```python
from build123d import *

# Parameters (mm, degrees)
F0_W     = 59.3015290797
F0_H     = 91.5408506989
F1_DEPTH = 47.752
F2_R     = 16.5566766108
F3_T     = -2.54


# Not quite as in the source:
# - a shell that OpenCascade refuses in one call is made with other operations: the cavity is built on its own and cut out


with BuildPart() as f1:
    # F0 (on Front) → F1 (new body)
    with BuildSketch(Plane.XZ):
        with Locations((-0.7059704512, -7.1773678064)):
            Rectangle(F0_W, F0_H)
    extrude(amount=F1_DEPTH)

    # F2
    f2_edges = [f1.edges().sort_by_distance(p)[0] for p in [
        (-30.356735, -23.876, 38.593058),
        (-30.356735, -23.876, -52.947793),
        (-30.356735, 0, -7.177368),
        (-30.356735, -47.752, -7.177368),
        (28.944794, -23.876, -52.947793),
        (-0.70597, 0, -52.947793),
        (-0.70597, -47.752, -52.947793),
        (28.944794, -23.876, 38.593058),
        (-0.70597, 0, 38.593058),
        (-0.70597, -47.752, 38.593058),
    ]]
    fillet(f2_edges, radius=F2_R)

    # F3: a shell. OpenCascade refuses it in one call, so the cavity is built on its own and cut out:
    # the body offset inwards by the wall thickness, plus a prism from it out through each open face.
    f3_core = offset(f1.part, amount=F3_T, mode=Mode.PRIVATE)
    f3_exits = [f3_core.faces().sort_by_distance(p)[0] for p in [
        (26.404794, -23.876, -7.177368),
    ]]
    add(f3_core, mode=Mode.SUBTRACT)
    extrude(f3_exits, amount=-F3_T, mode=Mode.SUBTRACT)


solid = f1.part
```
The model under review builds one solid part; all positions refer to its coordinate system, in mm. A direction names the side the tool comes from. Round coordinates to 2 decimals unless told otherwise and drop trailing zeros. Loops run counter-clockwise (first coordinate to the right, second up) from the corner with the lowest first, then second, coordinate; pieces in that order, holes last. Notation, with made-up numbers: M 57.5,-24 L 86.5,-24 A27 ccw 86.5,0 Z; hole C 32,-31 d3. An arc over 180 degrees is marked long. Put each result on its own line as item: value.
Q1. To check wall thickness, follow L1, parallel to Y at x = 12.5, z = 19; L2, parallel to Y at x = -4, z = -37; L3, parallel to Z at x = 17, y = -19. State the ranges of each line that lie inside material, in increasing order.
Result set:
L1: y = -47.75 to -45.21, -2.54 to 0
L2: y = -47.74 to -45.2, -2.55 to -0.01
L3: z = -52.29 to -49.63, 35.27 to 37.94
Q2. Machinability: for faces 4 (the flat face through (-30.357, -24, -8)), 5 (the flat face through (28, -24, -36.391)), 6 (the cylindrical face through (6.58, -41, -46.41)), which of the approach directions +Z, -Z, +X, -X, +Y, -Y give a long, thin tool a straight path to every point of the face, cutting with its end or side? Answer none if there is none.
Result set:
face 4: +Z, -Z, -X, +Y, -Y
face 5: +X
face 6: none
Q3. For pin 1 (21.5 mm diameter, centred on x = 12, z = -0.5, fed in from +Y); pin 2 (11.5 mm diameter, centred on y = -26.5, z = -4.5, fed in from +X); pin 3 (5 mm diameter, centred on x = -20.5, z = -15.5, fed in from +Y); pin 4 (1.5 mm diameter, centred on x = 9, y = -5.5, fed in from +Z), all flat-tipped, find the tip position at first contact; note any pin that passes through.
Result set:
pin 1: stops at y = 0
pin 2: stops at x = -27.78
pin 3: stops at y = -0.54
pin 4: stops at z = 34.99
Q4. Consider section B-B, the plane y = -29. Give the boundary of the cut face in (x, z).
Result set:
outline: M -30.36,-36.39 A16.56 ccw -13.8,-52.95 L 12.39,-52.95 A16.56 ccw 28.94,-36.39 L 26.4,-36.39 A14.02 cw 12.39,-50.41 L -13.8,-50.41 A14.02 cw -27.82,-36.39 L -27.82,22.04 A14.02 cw -13.8,36.05 L 12.39,36.05 A14.02 cw 26.4,22.04 L 28.94,22.04 A16.56 ccw 12.39,38.59 L -13.8,38.59 A16.56 ccw -30.36,22.04 Z
Q5. Consider section A-A, the plane z = 12. Give the boundary of the cut face in (x, y).
Result set:
outline: M -30.36,-31.2 A16.56 ccw -13.8,-47.75 L 28.94,-47.75 L 28.94,-45.21 L -13.8,-45.21 A14.02 cw -27.82,-31.2 L -27.82,-16.56 A14.02 cw -13.8,-2.54 L 28.94,-2.54 L 28.94,0 L -13.8,0 A16.56 ccw -30.36,-16.56 Z
Q6. Consider section D-D, the plane z = 32.5. Give the boundary of the cut face in (x, y).
Result set:
outline: M -26.63,-31.2 A12.83 ccw -13.8,-44.03 L 25.22,-44.03 L 25.22,-3.73 L -13.8,-3.73 A12.83 ccw -26.63,-16.56 Z; hole M -23.13,-31.2 A9.33 ccw -13.8,-40.52 L 21.71,-40.52 L 21.71,-7.23 L -13.8,-7.23 A9.33 ccw -23.13,-16.56 Z
Q7. Consider section C-C, the plane x = -8.5. Give the boundary of the cut face in (y, z).
Result set:
outline: M -47.75,-36.39 A16.56 ccw -31.2,-52.95 L -16.56,-52.95 A16.56 ccw 0,-36.39 L 0,22.04 A16.56 ccw -16.56,38.59 L -31.2,38.59 A16.56 ccw -47.75,22.04 Z; hole M -45.21,-36.39 A14.02 ccw -31.2,-50.41 L -16.56,-50.41 A14.02 ccw -2.54,-36.39 L -2.54,22.04 A14.02 ccw -16.56,36.05 L -31.2,36.05 A14.02 ccw -45.21,22.04 Z
Q8. Mouldability with a two-part tool opening along X and no side actions: class faces 1 (the cylindrical face through (6.6, -6.8, 32.1)), 2 (the flat face through (7, -45.212, -8)), 3 (the cylindrical face through (-25.635, -4.979, -6.768)) as released by +X, released by -X, zero draft, split by the parting line, or undercut.
Result set:
face 1: undercut
face 2: zero draft
face 3: released by -X
